Source: CAD feature listing. Evaluate the final solid. Frame: model axes, mm. Face numbers are marked on the shaded views. Give positions to 0.01 mm unless a question says otherwise; leave off trailing zeros. Loops run counter-clockwise (first coordinate to the right, second up) from the corner with the lowest first, then second, coordinate; pieces in that order, holes last. Notation, with made-up numbers: (-10, 65) -> (-4, 65) arc R9 cw to (-4, 81) -> close; hole circle Ø1 at (15, 61.5). An arc over 180 degrees is marked (long way). Return JSON: item names as keys, results as strings. Group by question number.
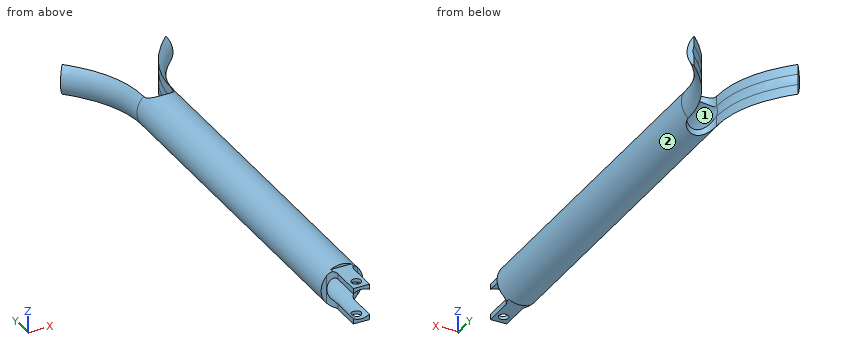
```python
from build123d import *

# Parameters (mm, degrees)
SKETCH1_R                = 1.0922
SKETCH1_R_2              = 0.7922
EXTRUDE_THIN1_DEPTH      = 20
SKETCH5_R                = 0.7422
CUT_EXTRUDE1_DEPTH       = 2.0922001
CUT_EXTRUDE1_DEPTH_BACK  = 2.0922001
CUT_EXTRUDE3_DEPTH       = 1
SKETCH10_W               = 7.629631572
SKETCH10_H               = 1.4248156
SKETCH10_H_2             = 1.107527322
CUT_EXTRUDE5_DEPTH       = 2
SKETCH9_R                = 0.25
CUT_EXTRUDE4_DEPTH       = 10
CUT_EXTRUDE4_DEPTH_BACK  = 10
CUT_EXTRUDE10_DEPTH      = 1.5
CUT_EXTRUDE10_DEPTH_BACK = 1.5


with BuildPart() as part:
    # Sketch1 → Extrude-Thin1 (new body)
    with BuildSketch(Plane(origin=(0, 0, 0), x_dir=(1, 0, 0), z_dir=(0, 1, 0))):
        Circle(SKETCH1_R)
        Circle(SKETCH1_R_2, mode=Mode.SUBTRACT)
    extrude(amount=EXTRUDE_THIN1_DEPTH)

    # Sweep1: sweep along a path in Sketch4
    with BuildLine(Plane.XY) as sweep1_path:
        add(Edge.make_bspline(
            [(-1.0922, 20), (-1.1, 22.819845093), (-4.0922, 25)],
            knots=[0, 0, 0, 1, 1, 1], degree=2))
    # Sketch3 → Sweep1 (sweep)
    with BuildSketch(Plane(origin=(0, 20, 0), x_dir=(1, 0, 0), z_dir=(0, 1, 0))):
        with BuildLine():
            Line((-0.7422, -0.276983754), (-0.7422, -0.801273986))
            ThreePointArc((-0.7422, -0.801273986), (-1.0922, 0), (-0.7422, 0.801273986))
            Line((-0.7422, 0.801273986), (-0.7422, 0.276983754))
            ThreePointArc((-0.7422, 0.276983754), (-0.7922, 0), (-0.7422, -0.276983754))
        make_face()
    sweep1 = sweep(path=sweep1_path.line)

    # Mirror1: Sweep1 across plane
    add(sweep1.mirror(Plane(origin=(0, 0, 0), x_dir=(0, 0, 1), z_dir=(1, 0, 0))))

    # Sketch5 → Cut-Extrude1 (cut, two sides)
    with BuildSketch(Plane.XY) as cut_extrude1_sk:
        with Locations((0, 20)):
            Circle(SKETCH5_R)
    extrude(amount=CUT_EXTRUDE1_DEPTH, mode=Mode.SUBTRACT)
    extrude(cut_extrude1_sk.sketch, amount=-CUT_EXTRUDE1_DEPTH_BACK, mode=Mode.SUBTRACT)

    # Sketch7 → Cut-Extrude3 (cut, symmetric)
    with BuildSketch(Plane.XY):
        Polygon((-3.943727123, 25.376725106), (-2.695468515, 24.323621974), (-3.002892381, 23.959227952), (-4.233358336, 24.997320174), align=None)
    cut_extrude3 = extrude(amount=CUT_EXTRUDE3_DEPTH, both=True, mode=Mode.SUBTRACT)

    # Mirror2: Cut-Extrude3 across plane
    add(cut_extrude3.mirror(Plane(origin=(0, 0, 0), x_dir=(0, 0, 1), z_dir=(1, 0, 0))), mode=Mode.SUBTRACT)

    # Sketch10 → Cut-Extrude5 (cut)
    with BuildSketch(Plane.XZ):
        with Locations((0.215570245, 1.6649078)):
            Rectangle(SKETCH10_W, SKETCH10_H)
        with Locations((0.215570245, -1.506263661)):
            Rectangle(SKETCH10_W, SKETCH10_H_2)
    extrude(amount=-CUT_EXTRUDE5_DEPTH, mode=Mode.SUBTRACT)

    # Sketch9 → Cut-Extrude4 (cut, two sides)
    with BuildSketch(Plane.XY) as cut_extrude4_sk:
        with Locations((0, 0.5)):
            Circle(SKETCH9_R)
    extrude(amount=CUT_EXTRUDE4_DEPTH, mode=Mode.SUBTRACT)
    extrude(cut_extrude4_sk.sketch, amount=-CUT_EXTRUDE4_DEPTH_BACK, mode=Mode.SUBTRACT)

    # Sketch11 → Cut-Extrude10 (cut, two sides)
    with BuildSketch(Plane.XY) as cut_extrude10_sk:
        with BuildLine():
            Line((0.425, 1.509625), (0.425, 0))
            Line((0.425, 0), (0.425, -2.073284984))
            Line((0.425, -2.073284984), (3.393193603, 1.9065))
            Line((3.393193603, 1.9065), (0.821875, 1.9065))
            ThreePointArc((0.821875, 1.9065), (0.541241996, 1.790258004), (0.425, 1.509625))
        make_face()
        with BuildLine():
            Line((-0.821875, 1.9065), (-3.393193603, 1.9065))
            Line((-3.393193603, 1.9065), (-0.425, -3.083793411))
            Line((-0.425, -3.083793411), (-0.425, 0))
            Line((-0.425, 0), (-0.425, 1.509625))
            ThreePointArc((-0.425, 1.509625), (-0.541241996, 1.790258004), (-0.821875, 1.9065))
        make_face()
    extrude(amount=CUT_EXTRUDE10_DEPTH, mode=Mode.SUBTRACT)
    extrude(cut_extrude10_sk.sketch, amount=-CUT_EXTRUDE10_DEPTH_BACK, mode=Mode.SUBTRACT)


solid = part.part
```
1) Contact query for flat-ended pins moving along their axis: P1, Ø1, axis at x = 0, z = 0, coming from the -Y side; P2, Ø0.9, axis at x = 0, y = 1, coming from the -Z side. Output: stop coordinate, or through.
2) Mould query, pull axis X, two halves, no side actions, for the marked faces 1 and 2. Classes: released by +X, released by -X, zero draft, split by the parting line, or undercut.
3) Cut plane C-C on y = 11.5. Return loops of the section in (x, z).
4) Material intervals for line 1 (Y direction, x = 0, z = 0.85); line 2 (X direction, y = 8.5, z = 0.05), sorted ascending.
5) Cut plane B-B on x = 0. Return loops of the section in (y, z), then the cut area to 3 significant figures.
6) Cut plane A-A on y = 0.5. Count the separate pieces of the cut face and the enclosed holes in it, then the cut area to 3 significant figures.
Calculated:
{
 "1": {"P1": "through", "P2": "z = -0.95"},
 "2": {"face 1": "undercut", "face 2": "split by the parting line"},
 "3": {"outline": "circle Ø2.18 at (0, 0); hole circle Ø1.58 at (0, 0)"},
 "4": {"line 1": "0 to 0.25, 0.75 to 19.26", "line 2": "-1.09 to -0.79, 0.79 to 1.09"},
 "5": {"outline": "(0, -0.95) -> (0.25, -0.95) -> (0.25, -0.79) -> (0, -0.79) -> close; (0, 0.79) -> (0.25, 0.79) -> (0.25, 0.95) -> (0, 0.95) -> close; (0.75, -0.95) -> (2, -0.95) -> (2, -1.09) -> (19.26, -1.09) -> (19.26, -0.79) -> (0.75, -0.79) -> close; (0.75, 0.79) -> (19.26, 0.79) -> (19.26, 1.09) -> (2, 1.09) -> (2, 0.95) -> (0.75, 0.95) -> close", "area": "10.8 mm2"},
 "6": {"separate pieces": "4", "enclosed holes": "0", "area": "0.167 mm2"}
}
